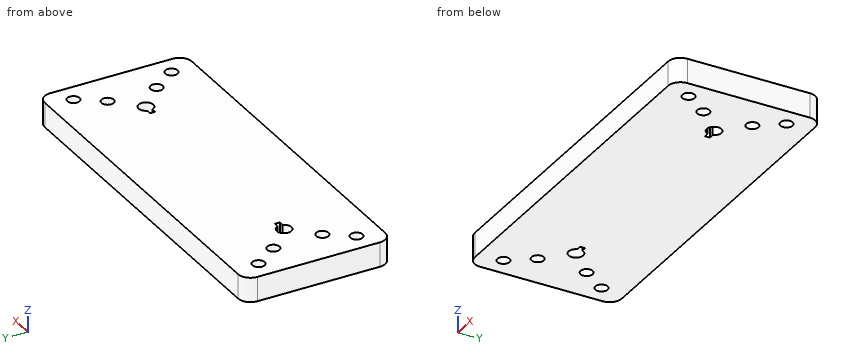
from build123d import *

# Parameters (mm, degrees)
BOSS_EXTRUDE1_DEPTH = 10
SKETCH2_R           = 2.5
CUT_EXTRUDE1_DEPTH  = 11
SKETCH3_R           = 2.5
CUT_EXTRUDE3_DEPTH  = 11


with BuildPart() as part:
    # Sketch1 → Boss-Extrude1 (new body)
    with BuildSketch(Plane.XY):
        with BuildLine():
            Line((5, 0), (145, 0))
            ThreePointArc((145, 0), (148.535533906, 1.464466094), (150, 5))
            Line((150, 5), (150, 55))
            ThreePointArc((150, 55), (148.535533906, 58.535533906), (145, 60))
            Line((145, 60), (5, 60))
            ThreePointArc((5, 60), (1.464466094, 58.535533906), (0, 55))
            Line((0, 55), (0, 5))
            ThreePointArc((0, 5), (1.464466094, 1.464466094), (5, 0))
        make_face()
        with BuildLine():
            Line((27.828427125, 31), (29.828427125, 31))
            Line((29.828427125, 31), (29.828427125, 29))
            Line((29.828427125, 29), (27.828427125, 29))
            ThreePointArc((27.828427125, 29), (22, 30), (27.828427125, 31))
        make_face(mode=Mode.SUBTRACT)
        with BuildLine():
            Line((122.171572875, 31), (120.171572875, 31))
            Line((120.171572875, 31), (120.171572875, 29))
            Line((120.171572875, 29), (122.171572875, 29))
            ThreePointArc((122.171572875, 29), (128, 30), (122.171572875, 31))
        make_face(mode=Mode.SUBTRACT)
    extrude(amount=BOSS_EXTRUDE1_DEPTH)

    # Sketch2 → Cut-Extrude1 (cut, through all)
    with BuildSketch(Plane.XY.offset(10)):
        with Locations((15, 40)):
            Circle(SKETCH2_R)
        with Locations((15, 20)):
            Circle(SKETCH2_R)
        with Locations((135, 40)):
            Circle(SKETCH2_R)
        with Locations((135, 20)):
            Circle(SKETCH2_R)
    extrude(amount=-CUT_EXTRUDE1_DEPTH, mode=Mode.SUBTRACT)

    # Sketch3 → Cut-Extrude3 (cut, through all)
    with BuildSketch(Plane.XY.offset(10)):
        with Locations((8, 50)):
            Circle(SKETCH3_R)
        with Locations((8, 10)):
            Circle(SKETCH3_R)
        with Locations((142, 50)):
            Circle(SKETCH3_R)
        with Locations((142, 10)):
            Circle(SKETCH3_R)
    extrude(amount=-CUT_EXTRUDE3_DEPTH, mode=Mode.SUBTRACT)


solid = part.part
Design review of the part built by this model. Coordinates are the model's own, in mm. Coordinates: 2 decimals unless noted, no trailing zeros. Order: outer loops, then holes, each group sorted by start corner. A loop starts at its lowest first (then second) coordinate and runs counter-clockwise, first axis right, second up. Notation, with made-up numbers: (-23.75, 60.5) -> (-5.75, 60.5) arc R17 ccw to (-5.75, 84.5) -> close; hole circle Ø2 at (51, 22). An arc over 180 degrees is marked (long way). Use one line per item in the form item = value. Start each with the question number.
(1) Add section D-D on z = 1.5. Give the number of separate pieces and of enclosed holes in the cut face, plus the area to 3 significant figures.
(2) Add section B-B on x = 25. State the section outline as (y, z) points, plus the area to 3 significant figures.
(3) Add section A-A on y = 50. State the section outline as (x, z) points, plus the area to 3 significant figures.
(4) Add section C-C on x = 142. State the section outline as (y, z) points.
(5) For probe 1 along Y at (x, z) = (15, 5.75); probe 2 along Y at (x, z) = (142, 7.5); probe 3 along X at (y, z) = (30, 5.5), list the stretches that pass through material, from the lowest coordinate up.
Answer block:
q1.separate_pieces = 1
q1.enclosed_holes = 10
q1.area = 8,760 mm²
q2.outline = (0, 0) -> (27, 0) -> (27, 10) -> (0, 10) -> close; (33, 0) -> (60, 0) -> (60, 10) -> (33, 10) -> close
q2.area = 540 mm²
q3.outline = (0, 0) -> (5.5, 0) -> (5.5, 10) -> (0, 10) -> close; (10.5, 0) -> (139.5, 0) -> (139.5, 10) -> (10.5, 10) -> close; (144.5, 0) -> (150, 0) -> (150, 10) -> (144.5, 10) -> close
q3.area = 1,400 mm²
q4.outline = (0, 0) -> (7.5, 0) -> (7.5, 10) -> (0, 10) -> close; (12.5, 0) -> (47.5, 0) -> (47.5, 10) -> (12.5, 10) -> close; (52.5, 0) -> (60, 0) -> (60, 10) -> (52.5, 10) -> close
q5.probe_1 = 0 to 17.5, 22.5 to 37.5, 42.5 to 60
q5.probe_2 = 0 to 7.5, 12.5 to 47.5, 52.5 to 60
q5.probe_3 = 0 to 22, 29.83 to 120.17, 128 to 150
